```python
from build123d import *

# Parameters (mm, degrees)
F0_R          = 4
F1_DEPTH      = 25
F0_W          = 3.3
F0_H          = 3.4
F4_DEPTH      = 15
F5_R          = 0.5
F6_DEPTH      = 26.4001190755
F6_DEPTH_BACK = 25


with BuildPart() as f1:
    # F0 (on Top) → F1 (new body)
    with BuildSketch(Plane.XY):
        Circle(F0_R)
        Polygon((-1.65, 3.4), (1.65, 3.4), (1.65, 0), (1.65, -3.4), (-1.65, -3.4), (-1.65, 0), align=None, mode=Mode.SUBTRACT)
    extrude(amount=F1_DEPTH)

    # F2 (on Front) → F3 (revolve)
    with BuildSketch(Plane.XZ):
        with BuildLine():
            Line((-24.7491189755, 0), (0, 0))
            Line((0, 0), (0, 10))
            Line((0, 10), (0, 11.2270785248))
            Line((0, 11.2270785248), (-12.3745594877, 10))
            add(Edge.make_bspline(
                [(-24.7491189755, 0), (-24.5552147878, 0.7300171854), (-23.7249598085, 5.3215287656), (-17.9770797483, 9.444446301), (-12.3745594877, 10)],
                knots=[0, 0, 0, 0, 0.3719475725, 1, 1, 1, 1], degree=3))
        make_face()
    revolve(axis=Axis((0, 0, 0), (0, 0, -1)))

    # F0 (on Top) → F4 (join)
    with BuildSketch(Plane.XY):
        with Locations((0, 1.7)):
            Rectangle(F0_W, F0_H)
        with Locations((0, -1.7)):
            Rectangle(F0_W, F0_H)
    extrude(amount=F4_DEPTH)

    # F5 (on face) → F6 (cut, two sides)
    with BuildSketch(Plane(origin=(1.65, 0, 0), x_dir=(0, -1, 0), z_dir=(-1, 0, 0))) as f6_sk:
        with Locations((0, 20)):
            Circle(F5_R)
    extrude(amount=F6_DEPTH, mode=Mode.SUBTRACT)
    extrude(f6_sk.sketch, amount=-F6_DEPTH_BACK, mode=Mode.SUBTRACT)


solid = f1.part
```
Read the model definition and answer for the solid it produces. Units are mm, in the model's axes. A direction names the side the tool comes from. Give positions to 0.01 mm unless a question says otherwise; leave off trailing zeros. Order: outer loops, then holes, each group sorted by start corner. A loop starts at its lowest first (then second) coordinate and runs counter-clockwise, first axis right, second up.
(1) For a pull along X with two mould halves and no side action, classify faces 3 (the flat face through (0, 0, 0)), 4 (the flat face through (-1.65, 1, 20)), 5 (the cylindrical face through (-0.867, -3.905, 17.816)) as released by +X, released by -X, zero draft, split by the parting line, or undercut.
(2) Given pin 1 (5.5 mm diameter, centred on y = 1.5, z = 18.5, fed in from -X); pin 2 (3.5 mm diameter, centred on x = -0.5, z = 20.5, fed in from -Y); pin 3 (10 mm diameter, centred on x = -18, z = 3.5, fed in from -Y), each flat-ended and moving along its own axis, determine where each tip first touches the part or whether it passes through.
(3) Straight lines are drawn through the part: L1, parallel to Z at x = 3, y = 0; L2, parallel to Y at x = 3.5, z = 20; L3, parallel to X at y = 1.5, z = 22. For each, find the intervals that lie inside material, in ascending order.
(4) Find section A-A (z = 14.25). Give the vertices of the cut face in (x, y).
(5) For faces 1 (the flat face through (2, 0, 25)), 2 (the flat face through (0, 0, 15)), determine the directions among +Z, -Z, +X, -X, +Y, -Y from which every point of the face is accessible in a straight line to the end or side of a thin tool.
Result sheet:
1. face 3: zero draft
1. face 4: undercut
1. face 5: split by the parting line
2. pin 1: stops at x = -4
2. pin 2: stops at y = -4
2. pin 3: stops at y = -20.34
3. L1: z = 0 to 19.5, 20.5 to 25
3. L2: y = -1.94 to -0.5, 0.5 to 1.94
3. L3: x = -3.71 to -1.65, 1.65 to 3.71
4. outline: circle Ø8 at (0, 0)
5. face 1: +Z, +X, -X, +Y, -Y
5. face 2: +Z
